Autodesk Fusion 360 part; units mm, degrees
sketch "Sketch1" plane through (0, 0, 0) normal (0, 0, 1) x (1, 0, 0)
  line L0 (12.5, -132.5) -> (-12.5, -132.5)
  line L1 (-12.5, -132.5) -> (-12.5, 132.5)
  line L2 (-12.5, 132.5) -> (12.5, 132.5)
  line L3 (12.5, 132.5) -> (12.5, -132.5)
  line L4 (12.5, -132.5) -> (-12.5, 132.5) construction
  line L5 (-12.5, -132.5) -> (12.5, 132.5) construction
  dimension "d1" = 25
  dimension "d2" = 265
extrude "Extrude1" add sketch "Sketch1" along normal blind 3
hole "Hole1" at (-2.5, 102.5, 3) direction (0, 0, -1) diameter 5 depth 65 tip angle 118
hole "Hole2" at (-2.5, -102.5, 3) direction (0, 0, -1) diameter 5 depth 65 tip angle 118
Verification items for the finished model (mm, model axes). Give positions to 0.01 mm unless a question says otherwise; leave off trailing zeros. Loops run counter-clockwise (first coordinate to the right, second up) from the corner with the lowest first, then second, coordinate; pieces in that order, holes last. Notation, with made-up numbers: M 56,54 L 77,54 A31 ccw 77,90 Z; hole C 48,89 d2. An arc over 180 degrees is marked long. Return JSON: item names as keys, results as strings.
1) Mould release check, pull along X, two halves, no side actions. Record for faces 1 (the cylindrical face through (-3.251, -104.885, 1.479)), 2 (the flat face through (0, 2, 3)): released by +X, released by -X, zero draft, split by the parting line, or undercut.
Findings:
{"face 1": "undercut", "face 2": "zero draft"}
2) Material ranges on L1, parallel to Y at x = -3, z = 1.3; L2, parallel to Y at x = -2.5, z = 1.65; L3, parallel to X at y = -102.5, z = 0.75, recorded low to high. Write a range as [from, to].
Findings:
{"L1": "y = [-132.5, -104.95], [-100.05, 100.05], [104.95, 132.5]", "L2": "y = [-132.5, -105], [-100, 100], [105, 132.5]", "L3": "x = [-12.5, -5], [0, 12.5]"}
3) Section check B-B, the plane y = -102.5. Enter the section's corners in (x, z), and give its area (3 significant figures).
Findings:
{"outline": "M -12.5,0 L -5,0 L -5,3 L -12.5,3 Z; M 0,0 L 12.5,0 L 12.5,3 L 0,3 Z", "area": "60.0 mm2"}
4) Section check A-A, the plane x = -2.5. Enter the section's corners in (y, z).
Findings:
{"outline": "M -132.5,0 L -105,0 L -105,3 L -132.5,3 Z; M -100,0 L 100,0 L 100,3 L -100,3 Z; M 105,0 L 132.5,0 L 132.5,3 L 105,3 Z"}
